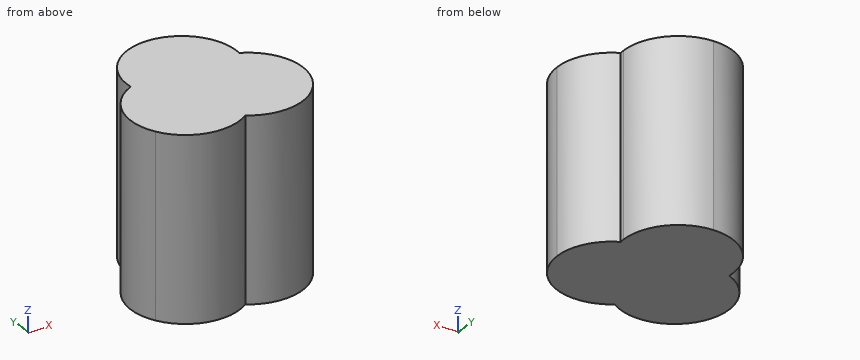
```python
from build123d import *

# Parameters (mm, degrees)
F1_DEPTH = 6


with BuildPart() as f1:
    # F0 (on Top) → F1 (new body)
    with BuildSketch(Plane.XY):
        with BuildLine():
            ThreePointArc((1.8, 1.2), (1.2727922061, 2.4727922061), (0, 3))
            ThreePointArc((0, 3), (-1.3299014134, 2.4129972096), (-1.7924074484, 1.0348469228))
            ThreePointArc((-1.7924074484, 1.0348469228), (-0.9565667293, 1.1981008602), (-0.1392304845, 0.9588457268))
            Line((-0.1392304845, 0.9588457268), (0, 1.2))
            Line((0, 1.2), (0.1392304845, 0.9588457268))
            ThreePointArc((0.1392304845, 0.9588457268), (0.9565667293, 1.1981008602), (1.7924074484, 1.0348469228))
            ThreePointArc((1.7924074484, 1.0348469228), (1.7981008602, 1.1173362447), (1.8, 1.2))
        make_face()
        with BuildLine():
            Line((0, 1.2), (-0.1392304845, 0.9588457268))
            ThreePointArc((-0.1392304845, 0.9588457268), (-0.0685911424, 0.9158691459), (0, 0.8696938457))
            ThreePointArc((0, 0.8696938457), (0.0685911424, 0.9158691459), (0.1392304845, 0.9588457268))
            Line((0.1392304845, 0.9588457268), (0, 1.2))
        make_face()
        with BuildLine():
            Line((0.5196152464, 0.2999999928), (0.1392304845, 0.9588457268))
            ThreePointArc((0.1392304845, 0.9588457268), (0.0685911424, 0.9158691459), (0, 0.8696938457))
            ThreePointArc((0, 0.8696938457), (0.2906709317, 0.6129972066), (0.5196152464, 0.2999999928))
        make_face()
        with BuildLine():
            ThreePointArc((-0.5196152407, 0.3000000027), (-0.6762066199, -0.0547701947), (-0.7531769639, -0.4348469228))
            ThreePointArc((-0.7531769639, -0.4348469228), (-0.3855356915, -0.5582270134), (0, -0.6))
            ThreePointArc((0, -0.6), (0.3855356915, -0.5582270134), (0.7531769639, -0.4348469228))
            ThreePointArc((0.7531769639, -0.4348469228), (0.6762066217, -0.0547702002), (0.5196152464, 0.2999999928))
            ThreePointArc((0.5196152464, 0.2999999928), (0.2906709317, 0.6129972066), (0, 0.8696938457))
            ThreePointArc((0, 0.8696938457), (-0.2906709278, 0.6129972108), (-0.5196152407, 0.3000000027))
        make_face()
        with BuildLine():
            ThreePointArc((0, 0.8696938457), (-0.0685911424, 0.9158691459), (-0.1392304845, 0.9588457268))
            Line((-0.1392304845, 0.9588457268), (-0.5196152407, 0.3000000027))
            ThreePointArc((-0.5196152407, 0.3000000027), (-0.2906709278, 0.6129972108), (0, 0.8696938457))
        make_face()
        with BuildLine():
            ThreePointArc((-0.1392304845, 0.9588457268), (-0.9565667293, 1.1981008602), (-1.7924074484, 1.0348469228))
            ThreePointArc((-1.7924074484, 1.0348469228), (-1.5158691459, 0.2293606579), (-0.9, -0.3588457268))
            Line((-0.9, -0.3588457268), (-0.5196152407, 0.3000000027))
            Line((-0.5196152407, 0.3000000027), (-0.1392304845, 0.9588457268))
        make_face()
        with BuildLine():
            ThreePointArc((0.9, -0.3588457268), (1.5158691459, 0.2293606579), (1.7924074484, 1.0348469228))
            ThreePointArc((1.7924074484, 1.0348469228), (0.9565667293, 1.1981008602), (0.1392304845, 0.9588457268))
            Line((0.1392304845, 0.9588457268), (0.5196152464, 0.2999999928))
            Line((0.5196152464, 0.2999999928), (0.9, -0.3588457268))
        make_face()
        with BuildLine():
            ThreePointArc((0, -2.0696938457), (1.4247662137, -2.3582270051), (2.5980762498, -1.4999999333))
            ThreePointArc((2.5980762498, -1.4999999333), (2.7778969818, -1.065874244), (2.8392304845, -0.6))
            ThreePointArc((2.8392304845, -0.6), (2.5550996304, 0.3706393421), (1.7924074484, 1.0348469228))
            ThreePointArc((1.7924074484, 1.0348469228), (1.5158691459, 0.2293606579), (0.9, -0.3588457268))
            Line((0.9, -0.3588457268), (1.0392304845, -0.6))
            Line((1.0392304845, -0.6), (0.7607695155, -0.6))
            ThreePointArc((0.7607695155, -0.6), (0.5593024166, -1.4274615181), (0, -2.0696938457))
        make_face()
        with BuildLine():
            ThreePointArc((0.7531769639, -0.4348469228), (0.8274615181, -0.3985329012), (0.9, -0.3588457268))
            Line((0.9, -0.3588457268), (0.5196152464, 0.2999999928))
            ThreePointArc((0.5196152464, 0.2999999928), (0.6762066217, -0.0547702002), (0.7531769639, -0.4348469228))
        make_face()
        with BuildLine():
            ThreePointArc((0.7531769639, -0.4348469228), (0.7588703757, -0.5173362447), (0.7607695155, -0.6))
            Line((0.7607695155, -0.6), (1.0392304845, -0.6))
            Line((1.0392304845, -0.6), (0.9, -0.3588457268))
            ThreePointArc((0.9, -0.3588457268), (0.8274615181, -0.3985329012), (0.7531769639, -0.4348469228))
        make_face()
        with BuildLine():
            Line((0, -0.6), (0.7607695155, -0.6))
            ThreePointArc((0.7607695155, -0.6), (0.7588703757, -0.5173362447), (0.7531769639, -0.4348469228))
            ThreePointArc((0.7531769639, -0.4348469228), (0.3855356915, -0.5582270134), (0, -0.6))
        make_face()
        with BuildLine():
            ThreePointArc((-0.7531769639, -0.4348469228), (-0.7588703757, -0.5173362447), (-0.7607695155, -0.6))
            Line((-0.7607695155, -0.6), (0, -0.6))
            ThreePointArc((0, -0.6), (-0.3855356915, -0.5582270134), (-0.7531769639, -0.4348469228))
        make_face()
        with BuildLine():
            ThreePointArc((-0.7531769639, -0.4348469228), (-0.8274615181, -0.3985329012), (-0.9, -0.3588457268))
            Line((-0.9, -0.3588457268), (-1.0392304845, -0.6))
            Line((-1.0392304845, -0.6), (-0.7607695155, -0.6))
            ThreePointArc((-0.7607695155, -0.6), (-0.7588703757, -0.5173362447), (-0.7531769639, -0.4348469228))
        make_face()
        with BuildLine():
            Line((-0.5196152407, 0.3000000027), (-0.9, -0.3588457268))
            ThreePointArc((-0.9, -0.3588457268), (-0.8274615181, -0.3985329012), (-0.7531769639, -0.4348469228))
            ThreePointArc((-0.7531769639, -0.4348469228), (-0.6762066199, -0.0547701947), (-0.5196152407, 0.3000000027))
        make_face()
        with BuildLine():
            ThreePointArc((-0.7607695155, -0.6), (-0.5593024166, -1.4274615181), (0, -2.0696938457))
            ThreePointArc((0, -2.0696938457), (0.5593024166, -1.4274615181), (0.7607695155, -0.6))
            Line((0.7607695155, -0.6), (0, -0.6))
            Line((0, -0.6), (-0.7607695155, -0.6))
        make_face()
        with BuildLine():
            ThreePointArc((-1.7924074484, 1.0348469228), (-2.7546675887, -0.0547701937), (-2.5980762141, -1.4999999953))
            ThreePointArc((-2.5980762141, -1.4999999953), (-1.4247661787, -2.3582270128), (0, -2.0696938457))
            ThreePointArc((0, -2.0696938457), (-0.5593024166, -1.4274615181), (-0.7607695155, -0.6))
            Line((-0.7607695155, -0.6), (-1.0392304845, -0.6))
            Line((-1.0392304845, -0.6), (-0.9, -0.3588457268))
            ThreePointArc((-0.9, -0.3588457268), (-1.5158691459, 0.2293606579), (-1.7924074484, 1.0348469228))
        make_face()
    extrude(amount=F1_DEPTH)


solid = f1.part
```
Geometry: final body of the model. Coordinates: model frame, mm. Round coordinates to 2 decimals unless told otherwise and drop trailing zeros. Loops run counter-clockwise (first coordinate to the right, second up) from the corner with the lowest first, then second, coordinate; pieces in that order, holes last.
Item 1: Section B-B, the plane x = 2.1. Output: boundary loops of the cut face in (y, z).
Checked values:
outline: (-2.05, 0) - (0.85, 0) - (0.85, 6) - (-2.05, 6) - close
Item 2: Contact query for a flat-ended pin moving along its axis: P1, Ø3, axis at x = -2, z = 1.5, coming from the +Y side. Output: stop coordinate, or through.
Checked values:
P1: stops at y = 2.93
Item 3: Line query: L1, parallel to X at y = 2.65, z = 0.8; L2, parallel to X at y = 2.3, z = 3.6; L3, parallel to Y at x = -1.35, z = 4.2. Output: solid intervals per line, ascending.
Checked values:
L1: x = -1.07 to 1.07
L2: x = -1.42 to 1.42
L3: y = -2.37 to 2.39
Item 4: Section C-C, the plane y = 2.65. Output: boundary loops of the cut face in (x, z), plus the area to 3 significant figures.
Checked values:
outline: (-1.07, 0) - (1.07, 0) - (1.07, 6) - (-1.07, 6) - close
area: 12.8 mm2
